Verification items for the finished model (mm, model axes). A direction names the side the tool comes from. Coordinates: 2 decimals unless noted, no trailing zeros. Order: outer loops, then holes, each group sorted by start corner. A loop starts at its lowest first (then second) coordinate and runs counter-clockwise, first axis right, second up.
Q1. Draft check along X on faces 4 (the cylindrical face through (-7.92, -6.08, 1.97)), 5 (the flat face through (34, -6, 8)), 6 (the flat face through (0, -7, 0)). Enter one of: pulls with the +X half, pulls with the -X half, needs draft (parallel to the pull), parting line crosses it, or undercut.
Q2. Thickness scan on line 1 (Y direction, x = 68, z = 7.9); line 2 (Y direction, x = 0.5, z = 1.5); line 3 (X direction, y = 3.5, z = 6.25). Record the ranges inside material, lowest first.
Q3. Cross-section at C-C, the plane x = 7.5. Record the boundary of the cut face in (y, z), and give its area (3 significant figures).
Q4. Set-up check for faces 1 (the cylindrical face through (47.5, 0.1, 7.5)), 2 (the flat face through (-9, 5, 4)), 3 (the flat face through (34, 19, 7)): record each of +Z, -Z, +X, -X, +Y, -Y from which the full face is reachable in a straight line by a thin tool's end or side.
Q5. Depth check by flat-ended pin: P1, Ø3, axis at y = -10, z = 5.5, coming from the -X side; P2, Ø2.5, axis at x = 68, y = -10, coming from the +Z side; P3, Ø1.5, axis at y = 7, z = 2, coming from the -X side; P4, Ø19, axis at x = 68, y = 0, coming from the -Z side. Enter the tip coordinate at first touch or a pass-through.
Q6. Cross-section at D-D, the plane x = -8. Record the boundary of the cut face in (y, z).
Q7. Cross-section at B-B, the plane y = 4. Record the boundary of the cut face in (x, z), and give its area (3 significant figures).
Q8. Cross-section at A-A, the plane x = 72.5. Record the boundary of the cut face in (y, z), and give its area (3 significant figures).
from build123d import *

# Parameters (mm, degrees)
SKETCH_1_R          = 9.985
EXTRUDE_1_DEPTH     = 4
SKETCH_2_R          = 11.5
EXTRUDE_2_DEPTH     = 2
SKETCH_3_R          = 19
EXTRUDE_3_DEPTH     = 3
SKETCH_4_R          = 6
CUT_EXTRUDE_1_DEPTH = 29.337254631
EXTRUDE_START       = -3
SKETCH_5_R          = 1.5
SKETCH_5_R_2        = 6
EXTRUDE_4_DEPTH     = 3
SKETCH_6_R          = 6
CUT_EXTRUDE_2_DEPTH = 90.504189846


with BuildPart() as part:
    # 草图1 → 凸台-拉伸1 (new body)
    with BuildSketch(Plane.XY):
        Circle(SKETCH_1_R)
    extrude(amount=EXTRUDE_1_DEPTH)

    # 草图2 → 凸台-拉伸2 (add)
    with BuildSketch(Plane.XY.offset(4)):
        Circle(SKETCH_2_R)
    extrude(amount=EXTRUDE_2_DEPTH)

    # 草图3 → 凸台-拉伸3 (add)
    with BuildSketch(Plane.XY.offset(6)):
        Circle(SKETCH_3_R)
    extrude(amount=EXTRUDE_3_DEPTH)

    # 草图4 → 切除-拉伸1 (cut, through all)
    with BuildSketch(Plane(origin=(0, 0, 0), x_dir=(-1, 0, 0), z_dir=(0, 0, -1))):
        Circle(SKETCH_4_R)
    extrude(amount=-CUT_EXTRUDE_1_DEPTH, mode=Mode.SUBTRACT)

    # 草图5 → 凸台-拉伸4 (add)
    # profile 1 of 2: a face of its own
    with BuildSketch(Plane.XY.offset(9).offset(EXTRUDE_START)):
        with BuildLine():
            Line((68, 19), (0, 19))
            ThreePointArc((0, 19), (13.435028843, 13.435028843), (19, 0))
            ThreePointArc((19, 0), (13.435028843, -13.435028843), (0, -19))
            Line((0, -19), (68, -19))
            ThreePointArc((68, -19), (49, 0), (68, 19))
        make_face()
    # profile 2 of 2: a face of its own
    with BuildSketch(Plane.XY.offset(9).offset(EXTRUDE_START)):
        with BuildLine():
            ThreePointArc((87, 0), (81.435028843, 13.435028843), (68, 19))
            ThreePointArc((68, 19), (49, 0), (68, -19))
            ThreePointArc((68, -19), (81.435028843, -13.435028843), (87, 0))
        make_face()
        with Locations((68, -10)):
            Circle(SKETCH_5_R, mode=Mode.SUBTRACT)
        with Locations((58, 0)):
            Circle(SKETCH_5_R, mode=Mode.SUBTRACT)
        with Locations((68, 0)):
            Circle(SKETCH_5_R_2, mode=Mode.SUBTRACT)
        with Locations((78, 0)):
            Circle(SKETCH_5_R, mode=Mode.SUBTRACT)
        with Locations((68, 10)):
            Circle(SKETCH_5_R, mode=Mode.SUBTRACT)
    extrude(amount=EXTRUDE_4_DEPTH)

    # 草图6 → 切除-拉伸2 (cut, through all)
    with BuildSketch(Plane.XY.offset(9)):
        with Locations((68, 0)):
            Circle(SKETCH_6_R)
        with BuildLine():
            Line((26.5, 6), (41.5, 6))
            ThreePointArc((41.5, 6), (47.5, 0), (41.5, -6))
            Line((41.5, -6), (26.5, -6))
            ThreePointArc((26.5, -6), (20.5, 0), (26.5, 6))
        make_face()
    extrude(amount=-CUT_EXTRUDE_2_DEPTH, mode=Mode.SUBTRACT)


solid = part.part
Check values:
1. face 4: parting line crosses it
1. face 5: undercut
1. face 6: needs draft
2. line 1: y = -19 to -11.5, -8.5 to -6, 6 to 8.5, 11.5 to 19
2. line 2: y = -9.97 to -5.98, 5.98 to 9.97
2. line 3: x = -18.67 to -4.87, 4.87 to 21.63, 46.37 to 63.13, 72.87 to 86.67
3. outline: (-19, 6) - (-8.72, 6) - (-8.72, 4) - (-6.59, 4) - (-6.59, 0) - (6.59, 0) - (6.59, 4) - (8.72, 4) - (8.72, 6) - (19, 6) - (19, 9) - (-19, 9) - close
3. area: 202 mm2
4. face 1: +Z, -Z
4. face 2: -Z
4. face 3: +Z, -Z, +X, -X, +Y
5. P1: stops at x = -16.95
5. P2: passes through
5. P3: stops at x = -7.79
5. P4: stops at z = 6
6. outline: (-17.23, 6) - (-8.26, 6) - (-8.26, 4) - (-5.97, 4) - (-5.97, 0) - (5.97, 0) - (5.97, 4) - (8.26, 4) - (8.26, 6) - (17.23, 6) - (17.23, 9) - (-17.23, 9) - close
7. outline: (-18.57, 6) - (-10.78, 6) - (-10.78, 4) - (-9.15, 4) - (-9.15, 0) - (-4.47, 0) - (-4.47, 9) - (-18.57, 9) - close; (4.47, 0) - (9.15, 0) - (9.15, 4) - (10.78, 4) - (10.78, 6) - (22.03, 6) - (22.03, 9) - (4.47, 9) - close; (45.97, 6) - (63.53, 6) - (63.53, 9) - (45.97, 9) - close; (72.47, 6) - (86.57, 6) - (86.57, 9) - (72.47, 9) - close
7. area: 253 mm2
8. outline: (-18.46, 6) - (-3.97, 6) - (-3.97, 9) - (-18.46, 9) - close; (3.97, 6) - (18.46, 6) - (18.46, 9) - (3.97, 9) - close
8. area: 86.9 mm2
